Job drawing, mm, ordinate dimensions from the low corner. One solid piece. Give positions to 0.01 mm unless a question says otherwise; leave off trailing zeros. Write each loop counter-clockwise with the first axis right and the second up, starting at its lowest first coordinate (ties: lowest second). Pieces come first, ordered by that corner, then holes. Notation, with made-up numbers: M -39.5,17.25 L -30.5,17.25 A5 cw -30.5,22.25 Z; hole C -5.5,32 d5. An arc over 180 degrees is marked long. Use CSV: the item, a comma, the result in double quotes. Start each with the question number.
Item 1: Cut at A-A (y = 53). List the corners of the cut face in (x, z).
Item 2: Drill centre lines: line 1 (Y direction, x = 5, z = 3.5); line 2 (Y direction, x = 49.5, z = 4.75); line 3 (X direction, y = 73, z = 6.25). Where is each one in solid material? Low to high. Write a range as [from, to].
Item 3: Cut at C-C (z = 2.25). List the corners of the cut face in (x, y).
Item 4: Cut at B-B (x = 51). List the corners of the cut face in (y, z).
Item 5: Mould opens along Y. For the marked faces 1, 2, 3 and 4 say: released by +Y, released by -Y, zero draft, split by the parting line, or undercut.
Item 6: Cut at D-D (y = 10). List the corners of the cut face in (x, z).
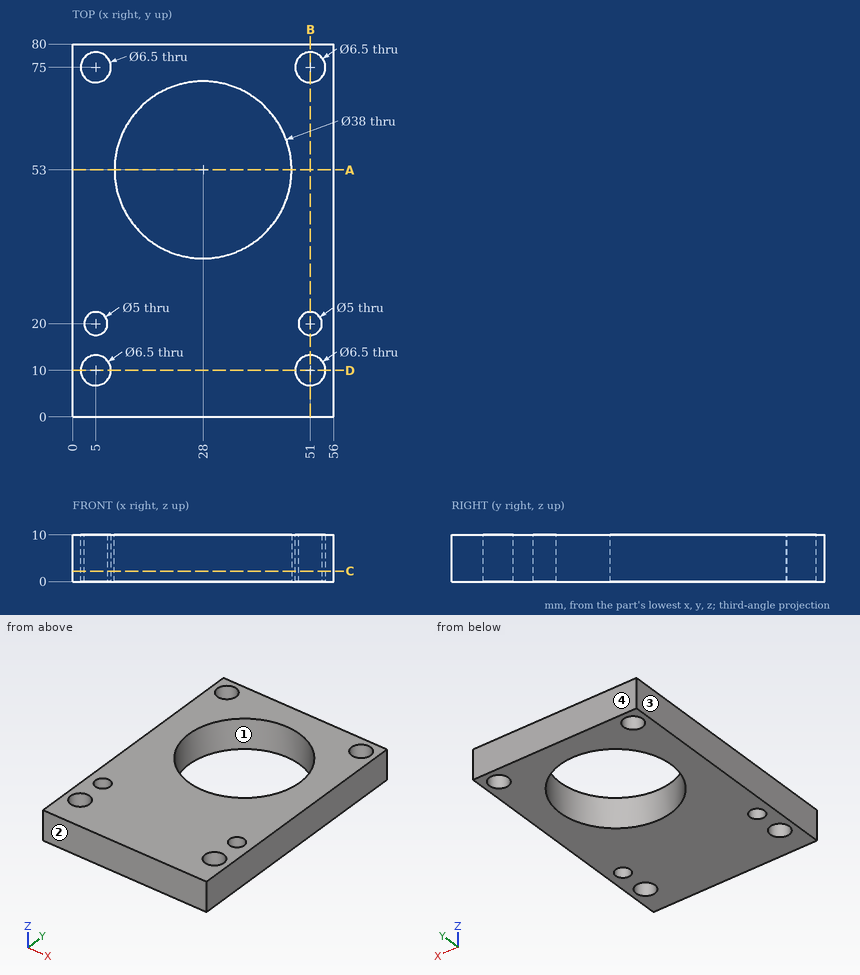
Worked answers:
1,outline,"M 0,0 L 9,0 L 9,10 L 0,10 Z; M 47,0 L 56,0 L 56,10 L 47,10 Z"
2,line 1,"y = [0, 6.75], [13.25, 17.5], [22.5, 71.75], [78.25, 80]"
2,line 2,"y = [0, 7.12], [12.88, 18], [22, 72.12], [77.88, 80]"
2,line 3,"x = [0, 2.44], [7.56, 48.44], [53.56, 56]"
3,outline,"M 0,0 L 56,0 L 56,80 L 0,80 Z; hole C 5,10 d6.5; hole C 5,75 d6.5; hole C 5,20 d5; hole C 28,53 d38; hole C 51,10 d6.5; hole C 51,75 d6.5; hole C 51,20 d5"
4,outline,"M 0,0 L 6.75,0 L 6.75,10 L 0,10 Z; M 13.25,0 L 17.5,0 L 17.5,10 L 13.25,10 Z; M 22.5,0 L 71.75,0 L 71.75,10 L 22.5,10 Z; M 78.25,0 L 80,0 L 80,10 L 78.25,10 Z"
5,face 1,"undercut"
5,face 2,"released by -Y"
5,face 3,"zero draft"
5,face 4,"released by +Y"
6,outline,"M 0,0 L 1.75,0 L 1.75,10 L 0,10 Z; M 8.25,0 L 47.75,0 L 47.75,10 L 8.25,10 Z; M 54.25,0 L 56,0 L 56,10 L 54.25,10 Z"
